Verification items for the finished model (mm, model axes). Face numbers are marked on the shaded views. A direction names the side the tool comes from. Coordinates: 2 decimals unless noted, no trailing zeros. Order: outer loops, then holes, each group sorted by start corner. A loop starts at its lowest first (then second) coordinate and runs counter-clockwise, first axis right, second up. Notation, with made-up numbers: M 77.25,26 L 92.25,26 A32 cw 92.25,57 Z; hole C 66.25,-6.5 d6. An arc over 180 degrees is marked long. Answer as a JSON object with one key per item and string values. Group by question number.
(1) Mould release check, pull along Z, two halves, no side actions. Record for the marked faces 1, 2 and 3: released by +Z, released by -Z, zero draft, split by the parting line, or undercut.
(2) Cross-section at C-C (y = 0.5). Enter the section's corners in (x, z).
(3) Gauge pin test, flat ends, axial feed: pin 1 Ø8 at (x, z) = (5.5, 6) entering from +Y; pin 2 Ø4 at (y, z) = (12, 3.5) entering from +X; pin 3 Ø4 at (x, z) = (-7.5, 6.5) entering from +Y. Record the tip position at first contact, or that the pin passes through.
(4) Access from +Z, -Z, +X, -X, +Y, -Y to the whole of each face (thin tool, end or side, straight path). Record for the marked faces 4, 5, 6 and 7.
(5) Cross-section at A-A (z = 12.5). Enter the section's corners in (x, y), plus the area to 3 significant figures.
(6) Material ranges on line 1 (Z direction, x = 5.5, y = 11); line 2 (Y direction, x = 0, z = 3.5) (3 decimals); line 3 (Y direction, x = 0, z = 12.5), recorded low to high.
(7) Cross-section at B-B (y = 13.5). Enter the section's corners in (x, z), plus the area to 3 significant figures.
from build123d import *

# Parameters (mm, degrees)
SKETCH1_R           = 15.875
BOSS_EXTRUDE1_DEPTH = 1
BOSS_EXTRUDE2_DEPTH = 10
SKETCH3_R           = 15.875
BOSS_EXTRUDE3_DEPTH = 1
SKETCH4_R           = 7
BOSS_EXTRUDE4_DEPTH = 5
CUT_EXTRUDE1_REACH  = 30.161
SKETCH5_R           = 3


with BuildPart() as part:
    # Sketch1 → Boss-Extrude1 (new body)
    with BuildSketch(Plane.XY):
        Circle(SKETCH1_R)
    extrude(amount=BOSS_EXTRUDE1_DEPTH)

    # Sketch2 → Boss-Extrude2 (add)
    with BuildSketch(Plane.XY.offset(1)):
        with BuildLine():
            Line((9.934806852, -4.423260993), (12.098542493, -4.403509345))
            ThreePointArc((12.098542493, -4.403509345), (12.376244335, -3.548830956), (12.593650359, -2.676863019))
            Line((12.593650359, -2.676863019), (10.769165248, -1.513507473))
            ThreePointArc((10.769165248, -1.513507473), (10.848509047, -0.758601652), (10.875, 0))
            Line((10.875, 0), (12.843637147, 0.898114599))
            ThreePointArc((12.843637147, 0.898114599), (12.749701385, 1.791853675), (12.593650359, 2.676863019))
            Line((12.593650359, 2.676863019), (10.453720943, 2.997556245))
            ThreePointArc((10.453720943, 2.997556245), (10.219157251, 3.719469059), (9.934806852, 4.423260993))
            Line((9.934806852, 4.423260993), (11.367950258, 6.044446371))
            ThreePointArc((11.367950258, 6.044446371), (10.918619238, 6.822710527), (10.416093803, 7.567735123))
            Line((10.416093803, 7.567735123), (8.330733319, 6.990315255))
            ThreePointArc((8.330733319, 6.990315255), (7.822820329, 7.554409779), (7.276795344, 8.081699977))
            Line((7.276795344, 8.081699977), (7.926641495, 10.145638453))
            ThreePointArc((7.926641495, 10.145638453), (7.199608632, 10.673858747), (6.4375, 11.150077074))
            Line((6.4375, 11.150077074), (4.767286221, 9.774385254))
            ThreePointArc((4.767286221, 9.774385254), (4.073846703, 10.083124418), (3.360559814, 10.342739615))
            Line((3.360559814, 10.342739615), (3.114744406, 12.492557476))
            ThreePointArc((3.114744406, 12.492557476), (2.235720287, 12.67939982), (1.345803965, 12.804469403))
            Line((1.345803965, 12.804469403), (0.379532027, 10.868375244))
            ThreePointArc((0.379532027, 10.868375244), (-0.379532027, 10.868375244), (-1.136747038, 10.815425612))
            Line((-1.136747038, 10.815425612), (-2.235720287, 12.67939982))
            ThreePointArc((-2.235720287, 12.67939982), (-3.114744406, 12.492557476), (-3.978593803, 12.244852647))
            Line((-3.978593803, 12.244852647), (-4.073846703, 10.083124418))
            ThreePointArc((-4.073846703, 10.083124418), (-4.767286221, 9.774385254), (-5.4375, 9.418026266))
            Line((-5.4375, 9.418026266), (-7.199608632, 10.673858747))
            ThreePointArc((-7.199608632, 10.673858747), (-7.926641495, 10.145638453), (-8.615056557, 9.567989628))
            Line((-8.615056557, 9.567989628), (-7.822820329, 7.554409779))
            ThreePointArc((-7.822820329, 7.554409779), (-8.330733319, 6.990315255), (-8.798059814, 6.392164619))
            Line((-8.798059814, 6.392164619), (-10.918619238, 6.822710527))
            ThreePointArc((-10.918619238, 6.822710527), (-11.367950258, 6.044446371), (-11.761897767, 5.23673428))
            Line((-11.761897767, 5.23673428), (-10.219157251, 3.719469059))
            ThreePointArc((-10.219157251, 3.719469059), (-10.453720943, 2.997556245), (-10.637355158, 2.261039638))
            Line((-10.637355158, 2.261039638), (-12.749701385, 1.791853675))
            ThreePointArc((-12.749701385, 1.791853675), (-12.843637147, 0.898114599), (-12.875, 0))
            Line((-12.875, 0), (-10.848509047, -0.758601652))
            ThreePointArc((-10.848509047, -0.758601652), (-10.769165248, -1.513507473), (-10.637355158, -2.261039638))
            Line((-10.637355158, -2.261039638), (-12.376244335, -3.548830956))
            ThreePointArc((-12.376244335, -3.548830956), (-12.098542493, -4.403509345), (-11.761897767, -5.23673428))
            Line((-11.761897767, -5.23673428), (-9.602055072, -5.105503245))
            ThreePointArc((-9.602055072, -5.105503245), (-9.222523046, -5.762871999), (-8.798059814, -6.392164619))
            Line((-8.798059814, -6.392164619), (-9.862822205, -8.275890475))
            ThreePointArc((-9.862822205, -8.275890475), (-9.261499929, -8.94372652), (-8.615056557, -9.567989628))
            Line((-8.615056557, -9.567989628), (-6.695318544, -8.569616945))
            ThreePointArc((-6.695318544, -8.569616945), (-6.081222825, -9.015783602), (-5.4375, -9.418026266))
            Line((-5.4375, -9.418026266), (-5.644028515, -11.571973346))
            ThreePointArc((-5.644028515, -11.571973346), (-4.82305989, -11.937492128), (-3.978593803, -12.244852647))
            Line((-3.978593803, -12.244852647), (-2.630900615, -10.551966023))
            ThreePointArc((-2.630900615, -10.551966023), (-1.888423932, -10.709784314), (-1.136747038, -10.815425612))
            Line((-1.136747038, -10.815425612), (-0.44933102, -12.867156898))
            ThreePointArc((-0.44933102, -12.867156898), (0.44933102, -12.867156898), (1.345803965, -12.804469403))
            Line((1.345803965, -12.804469403), (1.888423932, -10.709784314))
            ThreePointArc((1.888423932, -10.709784314), (2.630900615, -10.551966023), (3.360559814, -10.342739615))
            Line((3.360559814, -10.342739615), (4.82305989, -11.937492128))
            ThreePointArc((4.82305989, -11.937492128), (5.644028515, -11.571973346), (6.4375, -11.150077074))
            Line((6.4375, -11.150077074), (6.081222825, -9.015783602))
            ThreePointArc((6.081222825, -9.015783602), (6.695318544, -8.569616945), (7.276795344, -8.081699977))
            Line((7.276795344, -8.081699977), (9.261499929, -8.94372652))
            ThreePointArc((9.261499929, -8.94372652), (9.862822205, -8.275890475), (10.416093803, -7.567735123))
            Line((10.416093803, -7.567735123), (9.222523046, -5.762871999))
            ThreePointArc((9.222523046, -5.762871999), (9.602055072, -5.105503245), (9.934806852, -4.423260993))
        make_face()
    extrude(amount=BOSS_EXTRUDE2_DEPTH)

    # Sketch3 → Boss-Extrude3 (add)
    with BuildSketch(Plane.XY.offset(11)):
        Circle(SKETCH3_R)
    extrude(amount=BOSS_EXTRUDE3_DEPTH)

    # Sketch4 → Boss-Extrude4 (add)
    with BuildSketch(Plane.XY.offset(12)):
        Circle(SKETCH4_R)
    extrude(amount=BOSS_EXTRUDE4_DEPTH)

    # Sketch5 → Cut-Extrude1 (cut, up to next)
    with BuildSketch(Plane.XY.offset(17), mode=Mode.PRIVATE) as cut_extrude1_sk1:
        Circle(SKETCH5_R)
    cut_extrude1_tool1 = extrude(cut_extrude1_sk1.sketch, amount=-CUT_EXTRUDE1_REACH, mode=Mode.PRIVATE) & part.part
    add(cut_extrude1_tool1.solids().sort_by_distance((0, 0, 17))[0], mode=Mode.SUBTRACT)


solid = part.part
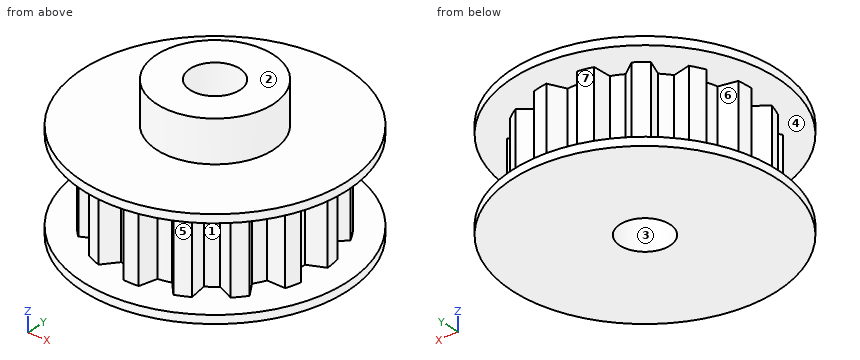
Taken from the geometry:
{
 "1": {"face 1": "undercut", "face 2": "released by +Z", "face 3": "zero draft"},
 "2": {"outline": "M -15.87,0 L -2.96,0 L -2.96,17 L -6.98,17 L -6.98,12 L -15.87,12 L -15.87,11 L -12.87,11 L -12.87,1 L -15.87,1 Z; M 2.96,0 L 15.87,0 L 15.87,1 L 11.97,1 L 11.97,11 L 15.87,11 L 15.87,12 L 6.98,12 L 6.98,17 L 2.96,17 Z"},
 "3": {"pin 1": "stops at y = 12.79", "pin 2": "stops at x = 7.93", "pin 3": "stops at y = 10.67"},
 "4": {"face 4": "none", "face 5": "+X, -Y", "face 6": "-X", "face 7": "-X, +Y"},
 "5": {"outline": "C 0,0 d14; hole C 0,0 d6", "area": "126 mm²"},
 "6": {"line 1": "z = 0 to 1, 11 to 12", "line 2": "y = -12.875 to -3, 3 to 10.875", "line 3": "y = -7 to -3, 3 to 7"},
 "7": {"outline": "M -8.35,0 L 8.35,0 L 8.35,1 L -8.35,1 Z; M -8.35,11 L 8.35,11 L 8.35,12 L -8.35,12 Z", "area": "33.4 mm²"}
}
